The listing builds one solid part. Answer for the finished solid, in the listing's coordinates (mm). A direction names the side the tool comes from. Coordinates: 2 decimals unless noted, no trailing zeros. Write each loop counter-clockwise with the first axis right and the second up, starting at its lowest first coordinate (ties: lowest second). Pieces come first, ordered by that corner, then holes.
(1) The part is cut by section A-A on x = 0. Determine the outline of the cut face in (y, z) (3 decimals).
(2) For a pull along Z with two mould halves and no side action, classify faces 1 (the cylindrical face through (0, 4, 5)), 2 (the flat face through (1.6, 5, 4.9)), 3 (the flat face through (2.788, 5.205, -0.021)) as +Z half, -Z half, draft (parallel to the pull), parting line (faces both ways), or undercut.
(3) Which of the six approach directions +Z, -Z, +X, -X, +Y, -Y give full straight-line access (tool end or side, diameter ignored) to faces 4 (the cylindrical face through (0, 4, -5)), 5 (the cylindrical face through (0.05, 4.644, 3.795)), 6 (the cylindrical face through (3, 5, 0)), 7 (the flat face through (4, 5.4, 0)), 8 (the conical face through (-0.054, 5.077, -3.954))?
(4) Straight lines are drawn through the part: line 1 (Y direction, x = -3, z = 4.5); line 2 (Z direction, x = 1.5, y = 3.85); line 3 (Z direction, x = -0.25, y = 4.75). For each, find the intervals that lie inside material, in ascending order.
(5) The part is cut by section B-B on y = 4.25. Determine the outline of the cut face in (x, z).
(6) The part is cut by section D-D on y = 5.15. Determine the outline of the cut face in (x, z).
(7) Given P1, Ø1.5, axis at x = 1.5, z = -2, coming from the +Y side, flat-ended and moving along its own axis, determine where the tip first touches the part or whether it passes through.
from build123d import *

# Parameters (mm, degrees)
SKETCH1_R               = 5
BOSS_EXTRUDE1_DEPTH     = 5
SKETCH2_R               = 5.5
BOSS_EXTRUDE2_DEPTH     = 0.4
CUT_EXTRUDE1_DEPTH      = 6.4
SKETCH5_R               = 8
CUT_EXTRUDE2_DEPTH      = 6.5
CUT_EXTRUDE2_DEPTH_BACK = 6.5
CHAMFER4_SIZE           = 1
CHAMFER4_SIZE2          = 0.383864035


with BuildPart() as part:
    # Sketch1 → Boss-Extrude1 (new body)
    with BuildSketch(Plane(origin=(0, 0, 0), x_dir=(1, 0, 0), z_dir=(0, 1, 0))):
        Circle(SKETCH1_R)
    extrude(amount=BOSS_EXTRUDE1_DEPTH)

    # Sketch2 → Boss-Extrude2 (add)
    with BuildSketch(Plane(origin=(0, 5, 0), x_dir=(1, 0, 0), z_dir=(0, 1, 0))):
        Circle(SKETCH2_R)
    extrude(amount=BOSS_EXTRUDE2_DEPTH)

    # Sketch4 → Cut-Extrude1 (cut, through all)
    with BuildSketch(Plane(origin=(0, 5.4, 0), x_dir=(1, 0, 0), z_dir=(0, 1, 0))):
        with BuildLine():
            Line((2.295250379, 1.5), (2.295250379, -1.5))
            ThreePointArc((2.295250379, -1.5), (0, -3.795250379), (-2.295250379, -1.5))
            Line((-2.295250379, -1.5), (-2.295250379, 1.5))
            ThreePointArc((-2.295250379, 1.5), (0, 3.795250379), (2.295250379, 1.5))
        make_face()
    extrude(amount=-CUT_EXTRUDE1_DEPTH, mode=Mode.SUBTRACT)

    # Sketch5 → Cut-Extrude2 (cut, two sides)
    with BuildSketch(Plane(origin=(0, 0, 0), x_dir=(0, 0, -1), z_dir=(1, 0, 0))) as cut_extrude2_sk:
        with Locations((0, -3)):
            Circle(SKETCH5_R)
    extrude(amount=CUT_EXTRUDE2_DEPTH, mode=Mode.SUBTRACT)
    extrude(cut_extrude2_sk.sketch, amount=-CUT_EXTRUDE2_DEPTH_BACK, mode=Mode.SUBTRACT)

    # Chamfer4
    chamfer4_edges = [part.edges().sort_by_distance(p)[0] for p in [
        (0, 5.4, -3.795250379),
        (-2.295250379, 5.4, 0),
        (0, 5.4, 3.795250379),
        (2.295250379, 5.4, 0),
    ]]
    chamfer4_side = [part.faces().sort_by_distance(p)[0] for p in [
        (-5.344436508, 5.4, 0),
    ]]
    chamfer(chamfer4_edges, length=CHAMFER4_SIZE, length2=CHAMFER4_SIZE2, reference=chamfer4_side[0])


solid = part.part
Model answer:
1. outline: (3.245, -5) - (5, -5) - (5, -5.5) - (5.4, -5.5) - (5.4, -4.795) - (5.016, -3.795) - (4.042, -3.795) arc R8 cw to start; (3.245, 5) arc R8 cw to (4.042, 3.795) - (5.016, 3.795) - (5.4, 4.795) - (5.4, 5.5) - (5, 5.5) - (5, 5) - close
2. face 1: +Z half
2. face 2: draft
2. face 3: undercut
3. face 4: -Z, -Y
3. face 5: +Y, -Y
3. face 6: +X, -X, -Y
3. face 7: +Z, -Z, +X, -X, +Y
3. face 8: +Y
4. line 1: y = 5 to 5.4
4. line 2: z = -4.77 to -4.13, 4.13 to 4.77
4. line 3: z = -4.99 to -3.78, 3.78 to 4.99
5. outline: (-3.68, -3.38) arc R5 ccw to (3.68, -3.38) - (1.31, -3.38) arc R2.3 cw to (-1.31, -3.38) - close; (-3.68, 3.38) - (-1.31, 3.38) arc R2.3 cw to (1.31, 3.38) - (3.68, 3.38) arc R5 ccw to start
6. outline: circle Ø11 at (0, 0); hole (-2.64, -1.5) arc R2.64 ccw to (2.64, -1.5) - (2.64, 1.5) arc R2.64 ccw to (-2.64, 1.5) - close
7. P1: stops at y = 5.03
